Read the model definition and answer for the solid it produces. Units are mm, in the model's axes. Face numbers are marked on the shaded views. A direction names the side the tool comes from. Give positions to 0.01 mm unless a question says otherwise; leave off trailing zeros. Loops run counter-clockwise (first coordinate to the right, second up) from the corner with the lowest first, then second, coordinate; pieces in that order, holes last. Notation, with made-up numbers: (13, 23) - (48, 23) arc R34 ccw to (48, 55) - close; hole circle Ø8 at (8.25, 82.5). An arc over 180 degrees is marked (long way). Write item = value, one per line.
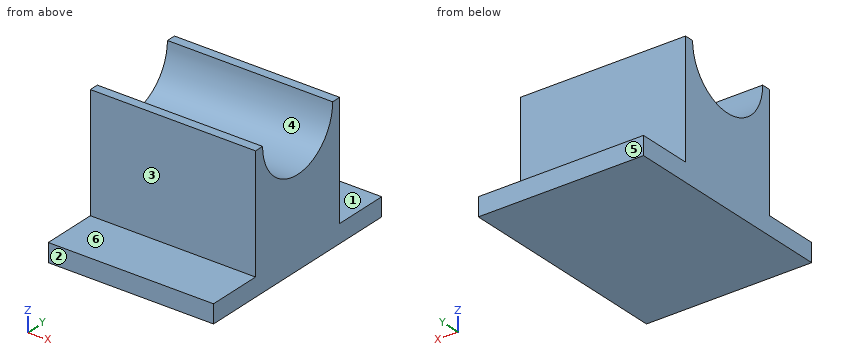
```python
from build123d import *

# Parameters (mm, degrees)
F1_DEPTH = 114.3
F3_DEPTH = 114.301


with BuildPart() as f1:
    # F0 (on Right) → F1 (new body)
    with BuildSketch(Plane.YZ):
        Polygon((0, 12.7), (0, 0), (152.4, 0), (152.4, 12.7), (114.3, 12.7), (114.3, 92.075), (38.1, 92.075), (38.1, 12.7), align=None)
    extrude(amount=F1_DEPTH)

    # F2 (on face) → F3 (cut, through all)
    with BuildSketch(Plane.YZ.offset(114.3)):
        with BuildLine():
            ThreePointArc((44.45, 92.075), (76.2, 60.325), (107.95, 92.075))
            Line((107.95, 92.075), (44.45, 92.075))
        make_face()
    extrude(amount=-F3_DEPTH, mode=Mode.SUBTRACT)


solid = f1.part
```
1) The mould has two halves that part along Y. Classify the marked faces 4, 5 and 6: pulls with the +Y half, pulls with the -Y half, needs draft (parallel to the pull), parting line crosses it, or undercut.
Output:
face_4 = undercut
face_5 = pulls with the +Y half
face_6 = needs draft
2) A cutting plane is placed at B-B on y = 76.2. Determine the outline of the cut face in (x, z) (3 decimals), then the cut area to 3 significant figures.
Output:
outline = (0, 0) - (114.3, 0) - (114.3, 60.325) - (0, 60.325) - close
area = 6,900 mm²
3) Each of these flat-tipped pins is pushed along its axis until it touches: P1, Ø6, axis at x = 48, y = 101, coming from the +Z side; P2, Ø19, axis at x = 82, y = 13, coming from the +Z side; P3, Ø8, axis at x = 39.5, z = 40, coming from the +Y side. Where does it stop, or does it pass through?
Output:
P1 = 76.74
P2 = 12.7
P3 = 114.3
4) A cutting plane is placed at A-A on x = 19. Determine the outline of the cut face in (y, z) (3 decimals).
Output:
outline = (0, 0) - (152.4, 0) - (152.4, 12.7) - (114.3, 12.7) - (114.3, 92.075) - (107.95, 92.075) arc R31.75 cw to (44.45, 92.075) - (38.1, 92.075) - (38.1, 12.7) - (0, 12.7) - close
5) A tool of negligible diameter and unlimited length cuts with its end or side. For the marked faces 1, 2 and 3, from which of +Z, -Z, +X, -X, +Y, -Y can it reach the whole face along a straight path? Write none if from no direction.
Output:
face_1 = +Z, +X, -X, +Y
face_2 = +Z, -Z, +X, -X, -Y
face_3 = +Z, +X, -X, -Y
6) Find the intervals of material crossed by probe 1 along Y at (x, z) = (107, 34); probe 2 along Z at (x, y) = (36, 11); probe 3 along Y at (x, z) = (69.5, 74.5), in increasing order.
Output:
probe_1 = 38.1 to 114.3
probe_2 = 0 to 12.7
probe_3 = 38.1 to 49.76, 102.64 to 114.3
7) A cutting plane is placed at C-C on z = 29. Determine the outline of the cut face in (x, y), then the cut area to 3 significant figures.
Output:
outline = (0, 38.1) - (114.3, 38.1) - (114.3, 114.3) - (0, 114.3) - close
area = 8,710 mm²
